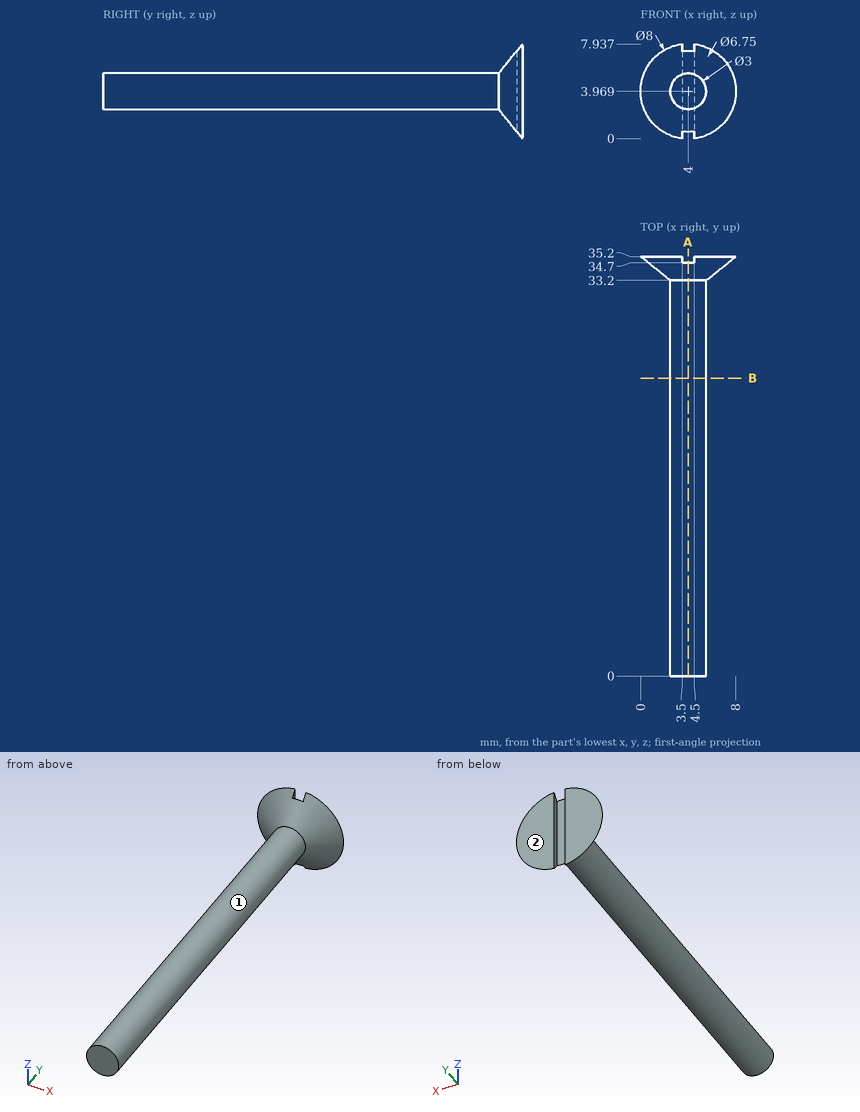
Check sheet for the drawn part. Datum: minimum x, y, z corner. Units: mm. A direction names the side the tool comes from. Coordinates: 2 decimals unless noted, no trailing zeros. Loops run counter-clockwise (first coordinate to the right, second up) from the corner with the lowest first, then second, coordinate; pieces in that order, holes last. Notation, with made-up numbers: (59.25, 66.25) - (72.25, 66.25) arc R29 cw to (72.25, 95.25) - close; hole circle Ø8 at (53.25, 67). An arc over 180 degrees is marked (long way). Put each result on its own line as item: value.
Item 1: Set-up check for the marked faces 1 and 2: record each of +Z, -Z, +X, -X, +Y, -Y from which the full face is reachable in a straight line by a thin tool's end or side.
Conclusion:
face 1: -Y
face 2: +Z, -Z, +X, -X, +Y
Item 2: Gauge pin test, flat ends, axial feed: pin 1 Ø0.6 at (y, z) = (35, 3) entering from +X; pin 2 Ø4 at (x, y) = (2, 31) entering from +Z; pin 3 Ø0.6 at (y, z) = (35, 2) entering from -X. Record the tip position at first contact, or that the pin passes through.
Conclusion:
pin 1: stops at x = 7.93
pin 2: stops at z = 5.47
pin 3: stops at x = 0.4
Item 3: Section check A-A (x = 4). Enter the section's corners in (y, z), then the cut area to 3 significant figures.
Conclusion:
outline: (0, 2.47) - (33.2, 2.47) - (34.7, 0.59) - (34.7, 7.34) - (33.2, 5.47) - (0, 5.47) - close
area: 107 mm2
Item 4: Section check B-B (y = 25). Enter the section's corners in (x, z).
Conclusion:
outline: circle Ø3 at (4, 3.97)
Item 5: Scan lines: line 1 along X through (y, z) = (28.5, 4); line 2 along Y through (x, z) = (1, 5.5) (1 decimal); line 3 along Y through (x, z) = (3, 1.25). Record each from-to range of solid material in increasing order.
Conclusion:
line 1: x = 2.5 to 5.5
line 2: y = 34.7 to 35.2
line 3: y = 34.32 to 35.2
